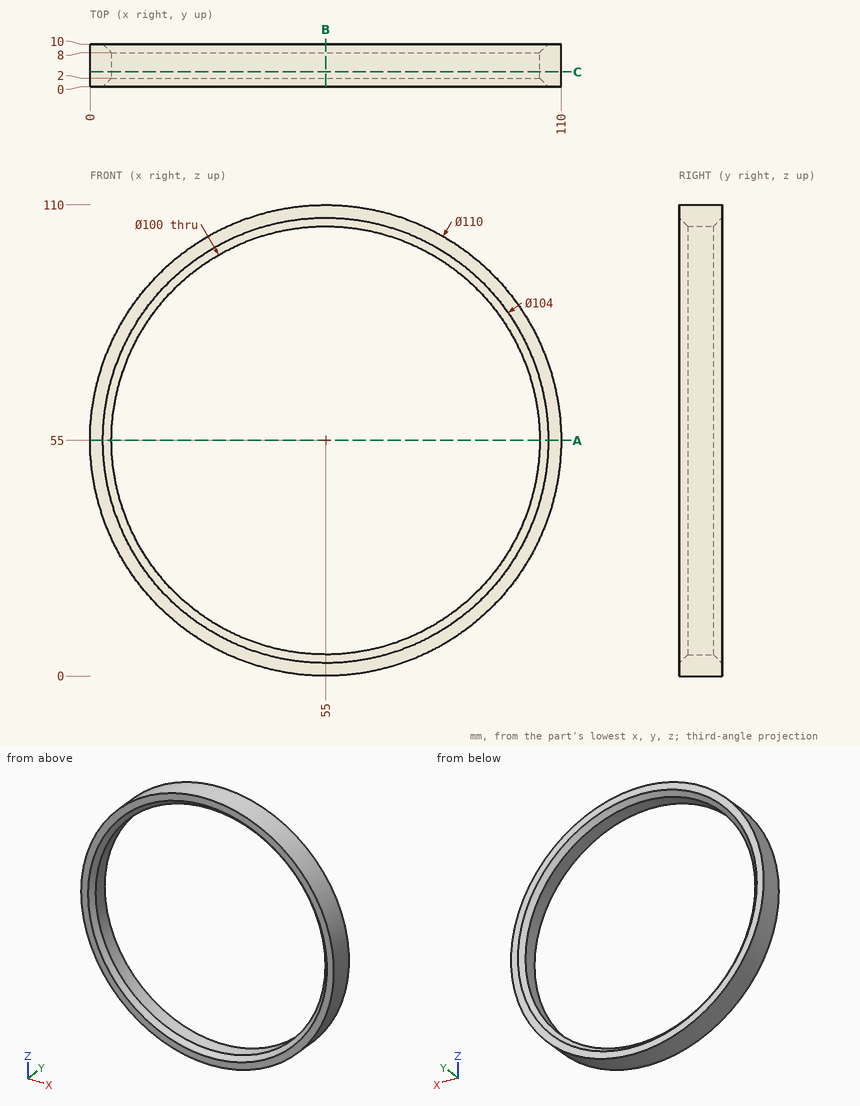
The drawing under review shows one solid part. Ordinate dimensions are in mm from its lowest x, y, z. Coordinates: 2 decimals unless noted, no trailing zeros. Order: outer loops, then holes, each group sorted by start corner. A loop starts at its lowest first (then second) coordinate and runs counter-clockwise, first axis right, second up. Notation, with made-up numbers: (-12, 63) -> (21, 63) arc R18 cw to (21, 85) -> close; hole circle Ø8 at (88, 87.5). An arc over 180 degrees is marked (long way). Answer in a Markdown table with one row per item.
(1) Consider section C-C (y = 3.5). Write out the cut boundary in (x, z), plus the area to 3 significant figures.
Answers:
| item | result |
|---|---|
| outline | circle Ø110 at (55, 55); hole circle Ø100 at (55, 55) |
| area | 1,650 mm² |
(2) Insertion check: pin 1 (1.5 mm diameter, centred on y = 6, z = 22, fed in from +X); pin 2 (1.5 mm diameter, centred on x = 93.5, y = 5, fed in from +Z); pin 3 (2 mm diameter, centred on y = 9, z = 14, fed in from +X). Each pin has a flat end and moves straight along its axis. Give the tip position at first contact, or say it passes through.
Answers:
| item | result |
|---|---|
| pin 1 | x = 99.55 |
| pin 2 | z = 95 |
| pin 3 | x = 92.75 |
(3) Consider section A-A (z = 55). Write out the cut boundary in (x, y).
Answers:
| item | result |
|---|---|
| outline | (0, 0) -> (3, 0) -> (5, 2) -> (5, 8) -> (3, 10) -> (0, 10) -> close; (105, 2) -> (107, 0) -> (110, 0) -> (110, 10) -> (107, 10) -> (105, 8) -> close |
(4) Consider section B-B (x = 55). Write out the cut boundary in (y, z).
Answers:
| item | result |
|---|---|
| outline | (0, 0) -> (10, 0) -> (10, 3) -> (8, 5) -> (2, 5) -> (0, 3) -> close; (0, 107) -> (2, 105) -> (8, 105) -> (10, 107) -> (10, 110) -> (0, 110) -> close |
(5) Wall thickness on line 1 along Z through (x, y) = (56.5, 6.25); line 2 along X through (y, z) = (9.75, 11); line 3 along X through (y, z) = (1, 97): over which ranges is each line inside the solid? List them lowest first.
Answers:
| item | result |
|---|---|
| line 1 | 0.02 to 5.02, 104.98 to 109.98 |
| line 2 | 22 to 27.76, 82.24 to 88 |
| line 3 | 19.49 to 26.07, 83.93 to 90.51 |
